Autodesk Fusion 360 part; units mm, degrees
sketch "Sketch1" plane through (0, 0, 0) normal (1, 0, 0) x (0, 0, -1)
  circle A0 centre (0, 0) radius 12.5
  line L0 (7.5, 7.5) -> (-7.5, 7.5)
  line L1 (-7.5, 7.5) -> (-7.5, -7.5)
  line L2 (-7.5, -7.5) -> (7.5, -7.5)
  line L3 (7.5, -7.5) -> (7.5, 7.5)
  line L4 (7.5, 7.5) -> (-7.5, -7.5) construction
  line L5 (-7.5, 7.5) -> (7.5, -7.5) construction
  dimension "d1" = 25
  dimension "d2" = 15
  dimension "d3" = 15
extrude "Extrude1" add sketch "Sketch1" along normal blind 8
sketch "Sketch2" plane through (0, 0, 0) normal (0, 1, 0) x (1, 0, 0)
sketch "Sketch3" plane through (8, 0, 0) normal (1, 0, 0) x (0, 0, -1)
  line L0 (7.5, 7.5) -> (7.5, -7.5)
  line L1 (7.5, -7.5) -> (-7.5, -7.5)
  line L2 (-7.5, -7.5) -> (-7.5, 7.5)
  line L3 (-7.5, 7.5) -> (7.5, 7.5)
  circle A0 centre (0, 0) radius 12.5
  line L4 (-5.7956, 9.4779) -> (6.4844, 9.4779)
  line L5 (6.4844, 9.4779) -> (-5.7956, 49.4779)
  line L6 (-5.7956, 49.4779) -> (-5.7956, 9.4779)
  dimension "d14" = 40
extrude "Extrude2" add sketch "Sketch3" along normal blind 2.5 from surface at -5 contours A0 L5 L6
sketch "Sketch4" plane through (0, 0, 0) normal (0, 1, 0) x (1, 0, 0)
  line L0 (2.9867, -5.8624) -> (5.5, -5.8624)
  line L1 (5.5, -5.8624) -> (5.5, 6)
  line L2 (5.5, 6) -> (2.9867, -5.8624)
extrude "Extrude3" cut sketch "Sketch4" against normal blind 39 from surface at 50
pattern_circular "C-Pattern1" count 4 over 360 about axis through (1.75, 0, 0) along (1, 0, 0) of "Extrude3", "Extrude2"
sketch "Sketch5" plane through (0, 0, 0) normal (0, 1, 0) x (-1, 0, 0)
sketch "Sketch6" plane through (8, 0, 0) normal (1, 0, 0) x (0, 0, -1)
  line L0 (7.5, 7.5) -> (7.5, -7.5)
  line L1 (7.5, -7.5) -> (-7.5, -7.5)
  line L2 (-7.5, -7.5) -> (-7.5, 7.5)
  line L3 (-7.5, 7.5) -> (7.5, 7.5)
  circle A0 centre (0, 0) radius 12.5
  circle A1 centre (0, 0) radius 12.5
  line L4 (7.5, 7.5) -> (-7.5, 7.5)
  line L5 (-7.5, 7.5) -> (-7.5, -7.5)
  line L6 (-7.5, -7.5) -> (7.5, -7.5)
  line L7 (7.5, -7.5) -> (7.5, 7.5)
  line L8 (7.5, 7.5) -> (-7.5, -7.5) construction
  line L9 (-7.5, 7.5) -> (7.5, -7.5) construction
extrude "Extrude4" add sketch "Sketch6" against normal blind 8
The listing builds one solid part. Answer for the finished solid, in the listing's coordinates (mm). A direction names the side the tool comes from. Give positions to 0.01 mm unless a question says otherwise; leave off trailing zeros. Loops run counter-clockwise (first coordinate to the right, second up) from the corner with the lowest first, then second, coordinate; pieces in that order, holes last.
Item 1: A cutting plane is placed at A-A (z = 2.5). Give the vertices of the cut face in (x, y).
Derived:
outline: (0, -12.25) - (3, -12.25) - (3, -22.46) - (5.5, -22.46) - (5.5, -12.25) - (8, -12.25) - (8, -7.5) - (0, -7.5) - close; (0, 7.5) - (8, 7.5) - (8, 12.25) - (3.7, 12.25) - (3.7, 38.74) - (3, 38.74) - (3, 12.25) - (0, 12.25) - close
Item 2: Determine the mould class of faces 6 (the flat face through (3.955, 25.662, -1.516)), 7 (the flat face through (4, 7.5, 0)), 8 (the flat face through (3, 22, 3)) for opening direction Z: +Z half, -Z half, draft (parallel to the pull), parting line (faces both ways), or undercut.
Derived:
face 6: -Z half
face 7: undercut
face 8: draft
Item 3: A cutting plane is placed at B-B (y = 0). Give the vertices of the cut face in (x, z), then the cut area to 3 significant figures.
Derived:
outline: (0, -12.5) - (3, -12.5) - (3, -30.6) - (5.5, -30.6) - (5.5, -12.5) - (8, -12.5) - (8, -7.5) - (0, -7.5) - close; (0, 7.5) - (8, 7.5) - (8, 12.5) - (5.5, 12.5) - (5.5, 30.6) - (3, 30.6) - (3, 12.5) - (0, 12.5) - close
area: 170 mm2
Item 4: A tool of negligible diameter and unlimited length cuts with its end or side. For faces 1 (the flat face through (0, -8, 0)), 2 (the cylindrical face through (3.94, -8.45, 9.21)), 3 (the flat face through (4, 5.796, -31)), 4 (the flat face through (4, -5.796, 31)), 5 (the flat face through (4, 0, -7.5)), from which of +Z, -Z, +X, -X, +Y, -Y can it reach the whole face along a straight path? Write none if from no direction.
Derived:
face 1: +Z, -Z, -X, +Y, -Y
face 2: none
face 3: -Z, +X, -X, +Y
face 4: +Z, +X, -X, -Y
face 5: +X, -X
Item 5: Each of these flat-tipped pins is pushed along its axis until it touches: pin 1 Ø1.5 at (x, z) = (3.5, 36.5) entering from -Y; pin 2 Ø3.5 at (y, z) = (1, 29) entering from +X; pin 3 Ø1.2 at (x, z) = (3.5, -39) entering from +Y. Where does it stop, or does it pass through?
Derived:
pin 1: stops at y = -5.8
pin 2: stops at x = 5.5
pin 3: stops at y = 5.8
Item 6: Find the intervals of material crossed by line 1 along X through (y, z) = (-3, 31.5); line 2 along Z through (x, y) = (7.75, 10); line 3 along Y through (x, z) = (6.5, -8.5), in increasing order.
Derived:
line 1: x = 3 to 5.5
line 2: z = -7.5 to 7.5
line 3: y = -9.17 to 9.17
Item 7: A cutting plane is placed at C-C (x = 4.25). Give the vertices of the cut face in (y, z).
Derived:
outline: (-49.48, -5.8) - (-11.08, -5.8) arc R12.5 ccw to (-6.03, -10.95) - (5.8, -49.48) - (5.8, -11.08) arc R12.5 ccw to (10.95, -6.03) - (30.27, -0.1) - (12.5, -0.1) arc R12.5 ccw to (6.03, 10.95) - (-5.8, 49.48) - (-5.8, 11.08) arc R12.5 ccw to (-10.95, 6.03) - close; hole (-7.5, -7.5) - (7.5, -7.5) - (7.5, 7.5) - (-7.5, 7.5) - close
